The model under review builds one solid part; all positions refer to its coordinate system, in mm. Round coordinates to 2 decimals unless told otherwise and drop trailing zeros. Write each loop counter-clockwise with the first axis right and the second up, starting at its lowest first coordinate (ties: lowest second). Pieces come first, ordered by that corner, then holes.
Item 1: Add section A-A (x = 75). Give the boundary of the cut face in (y, z), plus the area to 3 significant figures.
Item 2: To check wall thickness, follow L1, parallel to Z at x = 67.5, y = 1.75; L2, parallel to Y at x = 145, z = 1.4; L3, parallel to X at y = 5.5, z = 28.5. State the ranges of each line that lie inside material, in increasing order.
Item 3: Add section B-B (z = 23.5). Give the boundary of the cut face in (x, y), plus the area to 3 significant figures.
Item 4: Clearance check with flat-ended pins moving along their axes: pin 1 Ø4 at (y, z) = (3, 16) entering from -X; pin 2 Ø1 at (y, z) = (2.5, 25.5) entering from -X; pin 3 Ø5 at (y, z) = (7, 11) entering from +X. State where each tip first meets the part, or that it passes through.
Item 5: Add section C-C (x = 121). Give the boundary of the cut face in (y, z), plus the area to 3 significant figures.
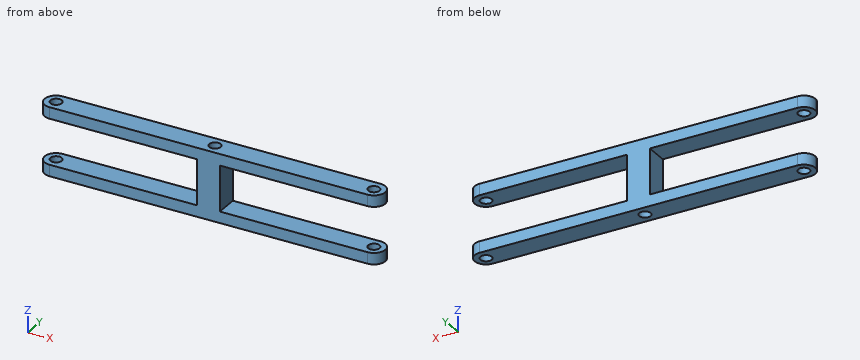
Autodesk Inventor part; units mm, degrees
ref_plane "YZ Plane" through (0, 0, 0) normal (1, 0, 0) x (0, 1, 0)
ref_plane "XZ Plane" through (0, 0, 0) normal (0, 1, 0) x (-1, 0, 0)
ref_plane "XY Plane" through (0, 0, 0) normal (0, 0, 1) x (1, 0, 0)
sketch "Sketch1" plane through (0, 0, 0) normal (0, 0, 1) x (1, 0, 0)
  line L0 (0, 0) -> (150, 0)
  line L1 (150, 0) -> (150, 10)
  line L2 (150, 10) -> (0, 10)
  line L3 (0, 10) -> (0, 0)
  circle A0 centre (5, 5) radius 2.5
  circle A1 centre (145, 5) radius 2.5
  dimension "d0" = 5
  dimension "d1" = 5
  dimension "d2" = 10
  dimension "d3" = 5
  dimension "d4" = 150
  dimension "d5" = 5
  dimension "d6" = 5
  dimension "d7" = 5
extrude "Extrusion1" add sketch "Sketch1" along normal blind 30
sketch "Sketch2" plane through (0, 10, 0) normal (0, 1, 0) x (1, 0, 0)
  point P0 (0, 0)
sketch "Sketch3" plane through (0, 10, 0) normal (0, 1, 0) x (1, 0, 0)
  line L0 (0, 0) -> (0, -30)
  line L1 (0, -25) -> (70, -25)
  line L2 (70, -25) -> (70, -5)
  line L3 (70, -5) -> (0, -5)
  line L4 (0, -5) -> (0, -25)
  line L5 (150, 0) -> (150, -30)
  line L6 (150, -25) -> (80, -25)
  line L7 (80, -25) -> (80, -5)
  line L8 (80, -5) -> (150, -5)
  line L9 (150, -5) -> (150, -25)
  line L10 (150, 0) -> (0, 0)
  line L11 (150, -30) -> (0, -30)
  point P0 (0, -5)
  dimension "d10" = 70
  dimension "d11" = 70
  dimension "d12" = 5
  dimension "d13" = 5
  dimension "d14" = 5
  dimension "d15" = 5
extrude "Extrusion2" cut sketch "Sketch3" against normal blind 10 contours L3 L2 L1 L0 | L5 L6 L7 L8
fillet "Fillet1" radius 5 8 edges at (0, 10, 27.5) (150, 10, 27.5) (150, 10, 2.5) (0, 10, 2.5) (150, 0, 27.5) (150, 0, 2.5) (0, 0, 27.5) (0, 0, 2.5)
sketch "Sketch4" plane through (0, 0, 30) normal (0, 0, 1) x (1, 0, 0)
  circle A0 centre (75, 5) radius 2.5
  line L0 (5, 0) -> (145, 0)
  circle A1 centre (5, 5) radius 2.5
  point P0 (0, 0)
  dimension "d19" = 5
  dimension "d20" = 5
  dimension "d21" = 70
extrude "Extrusion3" cut sketch "Sketch4" against normal blind 30 contours A0
properties part number "Joint 1"
Numbers:
1. outline: (0, 0) - (2.5, 0) - (2.5, 30) - (0, 30) - close; (7.5, 0) - (10, 0) - (10, 30) - (7.5, 30) - close
1. area: 150 mm2
2. L1: z = 0 to 5, 25 to 30
2. L2: y = 0 to 2.5, 7.5 to 10
2. L3: x = 0.03 to 2.55, 7.45 to 72.55, 77.45 to 142.55, 147.45 to 149.97
3. outline: (70, 0) - (80, 0) - (80, 10) - (70, 10) - close; hole circle Ø5 at (75, 5)
3. area: 80.4 mm2
4. pin 1: stops at x = 70
4. pin 2: stops at x = 0.42
4. pin 3: stops at x = 80
5. outline: (0, 0) - (10, 0) - (10, 5) - (0, 5) - close; (0, 25) - (10, 25) - (10, 30) - (0, 30) - close
5. area: 100 mm2
